Could you check a few things on this drawing? It's one solid part, dimensions in mm from its lowest x, y, z. Coordinates: 2 decimals unless noted, no trailing zeros. Loops run counter-clockwise (first coordinate to the right, second up) from the corner with the lowest first, then second, coordinate; pieces in that order, holes last.
1) Will these pins go through, and if not, where does the flat tip stop? P1, Ø3, axis at x = 46.4, y = 2.6, coming from the -Z side; P2, Ø2.5, axis at x = 46.4, y = 32.4, coming from the -Z side.
2) Imagine slicing it at A-A on y = 32.4. Please give me the cut outline in (x, z).
3) Imagine slicing it at C-C on z = 1.9. Please give me the cut outline in (x, y), plus the area to 3 significant figures.
4) If I drill on line 1 along Y through (x, z) = (46.4, 1.35); line 2 along Y through (x, z) = (2, 0.55); line 3 along X through (y, z) = (33, 1.65), over which ranges is the centre line in solid material (lowest first)?
5) Imagine slicing it at B-B on x = 24.5. Please give me the cut outline in (y, z).
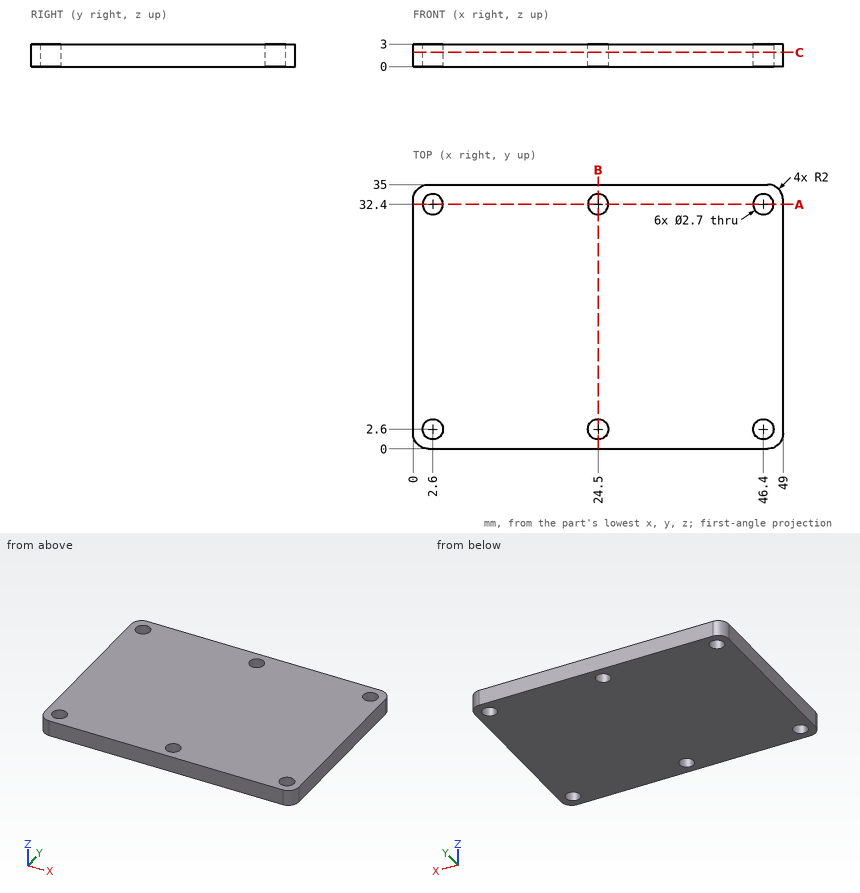
Filled in:
1. P1: stops at z = 0
1. P2: passes through
2. outline: (0, 0) - (1.25, 0) - (1.25, 3) - (0, 3) - close; (3.95, 0) - (23.15, 0) - (23.15, 3) - (3.95, 3) - close; (25.85, 0) - (45.05, 0) - (45.05, 3) - (25.85, 3) - close; (47.75, 0) - (49, 0) - (49, 3) - (47.75, 3) - close
3. outline: (0, 2) arc R2 ccw to (2, 0) - (47, 0) arc R2 ccw to (49, 2) - (49, 33) arc R2 ccw to (47, 35) - (2, 35) arc R2 ccw to (0, 33) - close; hole circle Ø2.7 at (2.6, 2.6); hole circle Ø2.7 at (2.6, 32.4); hole circle Ø2.7 at (24.5, 2.6); hole circle Ø2.7 at (24.5, 32.4); hole circle Ø2.7 at (46.4, 2.6); hole circle Ø2.7 at (46.4, 32.4)
3. area: 1,680 mm2
4. line 1: y = 0 to 1.25, 3.95 to 31.05, 33.75 to 35
4. line 2: y = 0 to 1.39, 3.81 to 31.19, 33.61 to 35
4. line 3: x = 0 to 1.39, 3.81 to 23.29, 25.71 to 45.19, 47.61 to 49
5. outline: (0, 0) - (1.25, 0) - (1.25, 3) - (0, 3) - close; (3.95, 0) - (31.05, 0) - (31.05, 3) - (3.95, 3) - close; (33.75, 0) - (35, 0) - (35, 3) - (33.75, 3) - close
